The listing builds one solid part. Answer for the finished solid, in the listing's coordinates (mm). Coordinates: 2 decimals unless noted, no trailing zeros. Order: outer loops, then holes, each group sorted by start corner. A loop starts at its lowest first (then second) coordinate and runs counter-clockwise, first axis right, second up. Notation, with made-up numbers: (-38.5, 67) -> (3.5, 67) arc R16 ccw to (3.5, 87) -> close; hole circle Ø4 at (8.5, -10.5). An arc over 180 degrees is marked (long way). Write item = value, one per line. Start each with the question number.
```python
from build123d import *

# Parameters (mm, degrees)
F0_W     = 7.2222218177
F0_H     = 63.1481452084
F1_DEPTH = 25
F0_W_2   = 10
F0_H_2   = 10
F0_W_3   = 24.2652441375
F0_H_3   = 6.617795676
F3_W     = 10
F3_H     = 14.9043388665
F4_DEPTH = 10
F5_R     = 5
F6_DEPTH = 25


with BuildPart() as f1:
    # F0 (on Front) → F1 (new body)
    with BuildSketch(Plane.XZ):
        with Locations((-45.9582116171, 0.8881576359)):
            Rectangle(F0_W, F0_H)
    extrude(amount=F1_DEPTH)

    # F3 (on Front) → F4 (join)
    with BuildSketch(Plane.XZ):
        Polygon((457.7808880806, 0), (-47.8088715536, 0), (-47.8088715536, -7), (467.7808880806, -7), (467.7808880806, 0), align=None)
        with Locations((462.7808880806, 7.4521694332)):
            Rectangle(F3_W, F3_H)
    extrude(amount=F4_DEPTH)

    # F5
    f5_edges = [f1.edges().sort_by_distance(p)[0] for p in [
        (457.780888, -5, 0),
        (467.780888, -5, -7),
    ]]
    fillet(f5_edges, radius=F5_R)

    # F6 (cut): a face of the model
    f6_faces = [f1.faces().sort_by_distance(p)[0] for p in [
        (-45.9582116171, -25, 0.8881576359),
    ]]
    extrude(f6_faces, amount=-F6_DEPTH, mode=Mode.SUBTRACT)


with BuildPart() as f1b:
    # F0 (on Front) → F1, piece 2 (new body)
    with BuildSketch(Plane.XZ):
        with Locations((462.6528992917, 20.9807503391)):
            Rectangle(F0_W_2, F0_H_2)
    extrude(amount=F1_DEPTH)


with BuildPart() as f1c:
    # F0 (on Front) → F1, piece 3 (new body)
    with BuildSketch(Plane.XZ):
        with Locations((19.7482968215, 31.2228444964)):
            Rectangle(F0_W_3, F0_H_3)
    extrude(amount=F1_DEPTH)


solid = f1.part
```
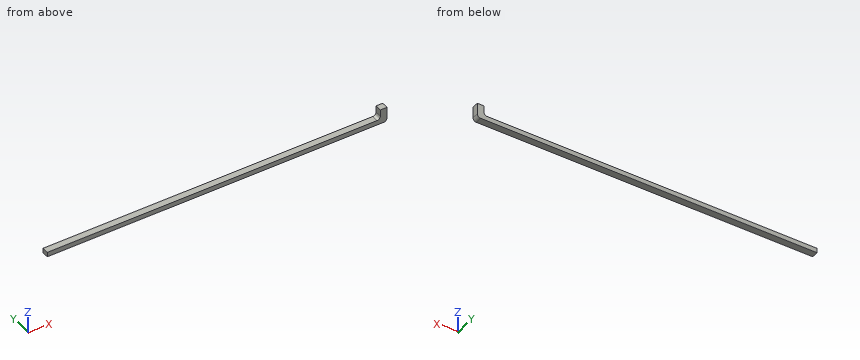
Item 1: Section A-A, the plane y = -3 is taken. Give the vertices of the cut face in (x, z).
Item 2: Section B-B, the plane x = 430 is taken. Give the vertices of the cut face in (y, z).
Item 3: Section C-C, the plane z = 11.25 is taken. Give the vertices of the cut face in (x, y), then the cut area to 3 significant figures.
Item 4: This flat-tipped pin is pushed along its axis until it touches: pin 1 (5 mm diameter, centred on y = -4, z = 10.5, fed in from -X). Where does it stop, or does it pass through?
Item 5: Consider probe 1 along Z at (x, y) = (178, -5.75); probe 2 along X at (y, z) = (-6, 11.5); probe 3 along X at (y, z) = (-3.5, 4). Determine where each line is inside the solid, lowest interval first.
A:
q1.outline = (-42.35, -7) -> (462.78, -7) arc R5 ccw to (467.78, -2) -> (467.78, 14.9) -> (457.78, 14.9) -> (457.78, 5) arc R5 cw to (452.78, 0) -> (-42.35, 0) -> close
q2.outline = (-10, -7) -> (0, -7) -> (0, 0) -> (-10, 0) -> close
q3.outline = (457.78, -10) -> (467.78, -10) -> (467.78, 0) -> (457.78, 0) -> close
q3.area = 100 mm^2
q4.pin_1 = 457.78
q5.probe_1 = -7 to 0
q5.probe_2 = 457.78 to 467.78
q5.probe_3 = 457.68 to 467.78
